Solid Edge part; units mm, degrees
sketch "Sketch1" plane through (0, 0, 0) normal (0, 0, 1) x (1, 0, 0)
  line L0 (50.5102, -49.2092) -> (-59.7414, -40.0215)
  line L1 (-59.7414, 39.9785) -> (-59.7414, -40.0215)
  line L2 (50.0837, 49.1305) -> (-59.7414, 39.9785)
  arc A0 (50.0837, 49.1305) -> (70.2586, 30.5669) centre (51.6306, 30.5669) cw
  line L3 (70.2586, -31.038) -> (70.2586, 30.5669)
  arc A1 (50.5102, -49.2092) -> (70.2586, -31.038) centre (52.0245, -31.038) ccw
  line L4 (16.6604, -50.4022) -> (-3.2705, -48.7413)
  line L5 (-3.2705, -48.7413) -> (-2.9383, -44.7551)
  line L6 (-2.9383, -44.7551) -> (16.9926, -46.4161)
  line L7 (16.9926, -46.4161) -> (16.6604, -50.4022)
  line L8 (-23.2014, -47.0804) -> (-43.1323, -45.4195)
  line L9 (-43.1323, -45.4195) -> (-42.8001, -41.4333)
  line L10 (-42.8001, -41.4333) -> (-22.8692, -43.0942)
  line L11 (-22.8692, -43.0942) -> (-23.2014, -47.0804)
  line L12 (-42.8001, 41.3902) -> (-22.8692, 43.0511)
  line L13 (-22.8692, 43.0511) -> (-23.2014, 47.0373)
  line L14 (-23.2014, 47.0373) -> (-43.1323, 45.3764)
  line L15 (-43.1323, 45.3764) -> (-42.8001, 41.3902)
  line L16 (16.6604, 50.3591) -> (-3.2705, 48.6982)
  line L17 (-3.2705, 48.6982) -> (-2.9383, 44.712)
  line L18 (-2.9383, 44.712) -> (16.9926, 46.373)
  line L19 (16.9926, 46.373) -> (16.6604, 50.3591)
  line L20 (-63.7414, 27.4785) -> (-63.7414, 7.4785)
  line L21 (-63.7414, 7.4785) -> (-59.7414, 7.4785)
  line L22 (-59.7414, 7.4785) -> (-59.7414, 27.4785)
  line L23 (-59.7414, 27.4785) -> (-63.7414, 27.4785)
  line L24 (-59.7414, -27.5215) -> (-59.7414, -7.5215)
  line L25 (-59.7414, -7.5215) -> (-63.7414, -7.5215)
  line L26 (-63.7414, -7.5215) -> (-63.7414, -27.5215)
  line L27 (-63.7414, -27.5215) -> (-59.7414, -27.5215)
  circle A2 centre (0.2586, 0) radius 2.5
extrude "Protrusion1" add sketch "Sketch1" along normal blind 4
Here's how the part is built. I have some questions about the finished solid (model axes, mm). A direction names the side the tool comes from. Give positions to 0.01 mm unless a question says otherwise; leave off trailing zeros. Loops run counter-clockwise (first coordinate to the right, second up) from the corner with the lowest first, then second, coordinate; pieces in that order, holes last. Notation, with made-up numbers: (78.5, -1) -> (87.5, -1) arc R35 ccw to (87.5, 38) -> close; hole circle Ø4 at (-19.5, -0.75). An arc over 180 degrees is marked (long way). One line per item, written item: value.
Q1. Suppose I cut it at C-C on x = -45.5. Please give me the cut outline in (y, z), then the cut area to 3 significant figures.
Answers follow:
outline: (-41.21, 0) -> (41.17, 0) -> (41.17, 4) -> (-41.21, 4) -> close
area: 329 mm^2
Q2. Suppose I cut it at A-A on y = 0. Please give me the cut outline in (x, z), then the cut area to 3 significant figures.
Answers follow:
outline: (-59.74, 0) -> (-2.24, 0) -> (-2.24, 4) -> (-59.74, 4) -> close; (2.76, 0) -> (70.26, 0) -> (70.26, 4) -> (2.76, 4) -> close
area: 500 mm^2
Q3. I'm going to push flat-ended pins straight in: pin 1 Ø1.2 at (y, z) = (-31, 2) entering from -X; pin 2 Ø2 at (x, z) = (-62, 2) entering from +Y; pin 3 Ø1.5 at (x, z) = (20, 3) entering from -Y. Where does each tip first touch, or does it pass through?
Answers follow:
pin 1: x = -59.74
pin 2: y = 27.48
pin 3: y = -46.73
Q4. On a 3-axis mill with a long thin cutter (end or side, diameter ignored), from which of +Z, -Z, +X, -X, +Y, -Y can I reach the whole of each face in a straight line? I mean faces 1 (the face through (16.83, -48.38, 1.97)), 2 (the face through (-59.741, -34, 2)), 3 (the face through (-42.97, 43.41, 1.97)), 4 (the face through (-3.107, -46.776, 1.972)). Say none if no direction works.
Answers follow:
face 1: +Z, -Z, -Y
face 2: +Z, -Z, -X, -Y
face 3: +Z, -Z, -X
face 4: +Z, -Z
Q5. If I drill on line 1 along X through (y, z) = (-31, 2.4); line 2 along Y through (x, z) = (-1, 1.75); line 3 along Y through (x, z) = (-7, 0.65), over which ranges is the centre line in solid material (lowest first)?
Answers follow:
line 1: -59.74 to 70.26
line 2: -48.93 to -2.16, 2.16 to 48.89
line 3: -44.42 to 44.37
Q6. Suppose I cut it at D-D on x = -31.5. Please give me the cut outline in (y, z), then the cut area to 3 significant figures.
Answers follow:
outline: (-46.39, 0) -> (46.35, 0) -> (46.35, 4) -> (-46.39, 4) -> close
area: 371 mm^2
Q7. We'd pull the mould along X, two halves only. Please class faces 5 (the face through (-23.033, -45.059, 1.972)), 6 (the face through (-51.152, -40.737, 1.972)), 7 (the face through (-62, 7.478, 2)): pulls with the +X half, pulls with the -X half, needs draft (parallel to the pull), parting line crosses it, or undercut.
Answers follow:
face 5: undercut
face 6: pulls with the -X half
face 7: needs draft
